from build123d import *

# Parameters (mm, degrees)
SKETCH1_W           = 53.5
SKETCH1_H           = 99
SKETCH1_R           = 1.666666667
BOSS_EXTRUDE1_DEPTH = 1.6
SKETCH2_W           = 46
SKETCH2_H           = 5
SKETCH2_W_2         = 2.4
SKETCH2_H_2         = 66.4
SKETCH2_H_3         = 70
SKETCH2_W_3         = 9
SKETCH2_H_4         = 14
SKETCH2_W_4         = 12.25
SKETCH2_H_5         = 16.5
BOSS_EXTRUDE2_DEPTH = 9


with BuildPart() as part:
    # Sketch1 → Boss-Extrude1 (new body)
    # profile 1 of 2: a face of its own
    with BuildSketch(Plane(origin=(0, 0, 0), x_dir=(1, 0, 0), z_dir=(0, 1, 0))):
        with Locations((26.75, 49.5)):
            Rectangle(SKETCH1_W, SKETCH1_H)
        with Locations(Location((50.833333333, 8.5, 0), (0, 0, 270))):
            Circle(SKETCH1_R, mode=Mode.SUBTRACT)
        with Locations(Location((2.666666667, 2.666666667, 0), (0, 0, 270))):
            Circle(SKETCH1_R, mode=Mode.SUBTRACT)
        with Locations(Location((36.083333333, 32.833333333, 0), (0, 0, 270))):
            Circle(SKETCH1_R, mode=Mode.SUBTRACT)
        with Locations(Location((7.666666667, 32.833333333, 0), (0, 0, 270))):
            Circle(SKETCH1_R, mode=Mode.SUBTRACT)
        with Locations(Location((50.833333333, 83.5, 0), (0, 0, 270))):
            Circle(SKETCH1_R, mode=Mode.SUBTRACT)
        with Locations(Location((2.666666667, 84.5, 0), (0, 0, 270))):
            Circle(SKETCH1_R, mode=Mode.SUBTRACT)
    # profile 2 of 2: a face of its own
    with BuildSketch(Plane(origin=(0, 0, 0), x_dir=(1, 0, 0), z_dir=(0, 1, 0))):
        Polygon((0, 0), (2.5, -2.5), (38, -2.5), (40.5, 0), align=None)
    extrude(amount=BOSS_EXTRUDE1_DEPTH)

    # Sketch2 → Boss-Extrude2 (add)
    with BuildSketch(Plane(origin=(0, 1.6, 0), x_dir=(1, 0, 0), z_dir=(0, 1, 0))):
        with Locations((29.22, 3.5)):
            Rectangle(SKETCH2_W, SKETCH2_H)
        with Locations((2.2, 38.8)):
            Rectangle(SKETCH2_W_2, SKETCH2_H_2)
        with Locations((51.3, 46)):
            Rectangle(SKETCH2_W_2, SKETCH2_H_3)
        with Locations((8.75, 93.63)):
            Rectangle(SKETCH2_W_3, SKETCH2_H_4)
        with Locations((38.465, 96.91)):
            Rectangle(SKETCH2_W_4, SKETCH2_H_5)
    extrude(amount=BOSS_EXTRUDE2_DEPTH)


solid = part.part
Check sheet for the modelled part. Datum: model origin and axes. Units: mm. A direction names the side the tool comes from. Coordinates: 2 decimals unless noted, no trailing zeros. Loops run counter-clockwise (first coordinate to the right, second up) from the corner with the lowest first, then second, coordinate; pieces in that order, holes last. Notation, with made-up numbers: (21.5, 16) -> (40.5, 16) arc R37 cw to (40.5, 55) -> close; hole circle Ø11 at (33.5, 15). An arc over 180 degrees is marked (long way). Write item = value, one per line. Start each with the question number.
1. Section check B-B on z = -8.5. Record the cut outline in (x, y).
2. Section check A-A on y = 6.75. Record the cut outline in (x, z), then the cut area to 3 significant figures.
3. Material ranges on line 1 (Z direction, x = 10, y = 9.25); line 2 (Z direction, x = 40, y = 5.75); line 3 (Z direction, x = 3, y = 1.5), recorded low to high.
4. Section check D-D on x = 21.5. Record the cut outline in (y, z), then the cut area to 3 significant figures.
5. Draft check along Z on faces 1 (the flat face through (29, 10.6, -4)), 2 (the cylindrical face through (37.736, 0.789, -33.05)), 3 (the flat face through (29, 6, -1)), 4 (the flat face through (38, 6, -105.16)). Enter one of: released by +Z, released by -Z, zero draft, split by the parting line, or undercut.
6. Tool access check on faces 5 (the flat face through (32.34, 6, -97)), 6 (the flat face through (4.25, 6, -94)), 7 (the flat face through (2, 6, -72)). Record the directions out of +Z, -Z, +X, -X, +Y, -Y that give a thin tool (end or side, any length) a straight path to the whole face; none if there is none.
7. Section check C-C on z = -97. Record the cut outline in (x, y), then the cut area to 3 significant figures.
8. Depth check by flat-ended pin: P1, Ø5.5, axis at y = 5.5, z = -3.5, coming from the -X side; P2, Ø3, axis at x = 2.67, z = -2.67, coming from the -Y side; P3, Ø6, axis at x = 13.5, z = -24.5, coming from the +Y side; P4, Ø4.5, axis at y = 8, z = -94, coming from the +X side. Enter the tip coordinate at first touch or a pass-through.
Responses:
q1.outline = (0, 0) -> (49.17, 0) -> (49.17, 1.6) -> (3.4, 1.6) -> (3.4, 10.6) -> (1, 10.6) -> (1, 1.6) -> (0, 1.6) -> close; (52.5, 0) -> (53.5, 0) -> (53.5, 1.6) -> (52.5, 1.6) -> close
q2.outline = (1, -72) -> (3.4, -72) -> (3.4, -5.6) -> (1, -5.6) -> close; (4.25, -100.63) -> (13.25, -100.63) -> (13.25, -86.63) -> (4.25, -86.63) -> close; (6.22, -6) -> (52.22, -6) -> (52.22, -1) -> (6.22, -1) -> close; (32.34, -105.16) -> (44.59, -105.16) -> (44.59, -88.66) -> (32.34, -88.66) -> close; (50.1, -81) -> (52.5, -81) -> (52.5, -11) -> (50.1, -11) -> close
q2.area = 885 mm2
q3.line_1 = -100.63 to -86.63, -6 to -1
q3.line_2 = -105.16 to -88.66, -6 to -1
q3.line_3 = -99 to -86.13, -82.87 to -4.3, -1.03 to 2.5
q4.outline = (0, -99) -> (1.6, -99) -> (1.6, -6) -> (10.6, -6) -> (10.6, -1) -> (1.6, -1) -> (1.6, 2.5) -> (0, 2.5) -> close
q4.area = 207 mm2
q5.face_1 = zero draft
q5.face_2 = undercut
q5.face_3 = released by +Z
q5.face_4 = released by -Z
q6.face_5 = -Z, +Y
q6.face_6 = +Z, -Z, -X, +Y
q6.face_7 = -Z, -X, +Y
q7.outline = (0, 0) -> (53.5, 0) -> (53.5, 1.6) -> (44.59, 1.6) -> (44.59, 10.6) -> (32.34, 10.6) -> (32.34, 1.6) -> (13.25, 1.6) -> (13.25, 10.6) -> (4.25, 10.6) -> (4.25, 1.6) -> (0, 1.6) -> close
q7.area = 277 mm2
q8.P1 = 1
q8.P2 = through
q8.P3 = 1.6
q8.P4 = 44.59
